Autodesk Inventor part; units mm, degrees
ref_plane "YZ Plane" through (0, 0, 0) normal (1, 0, 0) x (0, 1, 0)
ref_plane "XZ Plane" through (0, 0, 0) normal (0, 1, 0) x (-1, 0, 0)
ref_plane "XY Plane" through (0, 0, 0) normal (0, 0, 1) x (1, 0, 0)
sketch "Sketch1" plane through (0, 0, 0) normal (1, 0, 0) x (0, 1, 0)
  line L0 (0, 18.823) -> (0, -81.823)
  line L1 (-50.323, 0) -> (13.573, 0)
  line L2 (0, 0) -> (0, -63)
  line L3 (0, -63) -> (-28, -63)
  line L4 (-28, -63) -> (-28, -24.33)
  line L5 (-28, -24.33) -> (-36.75, -24.33)
  line L6 (-36.75, -24.33) -> (-36.75, 0)
  line L7 (-36.75, 0) -> (0, 0)
  circle A0 centre (-16, -42.5) radius 1.575 construction
  line L8 (-35.988, -0.762) -> (-35.988, -23.568)
  line L9 (-35.988, -23.568) -> (-27.238, -23.568)
  line L10 (-27.238, -23.568) -> (-27.238, -62.238)
  line L11 (-27.238, -62.238) -> (-0.762, -62.238)
  line L12 (-0.762, -62.238) -> (-0.762, -0.762)
  line L13 (-0.762, -0.762) -> (-35.988, -0.762)
  line L14 (-41.195, 4.445) -> (-41.195, -28.775)
  line L15 (-41.195, -28.775) -> (-32.445, -28.775)
  line L16 (-32.445, -28.775) -> (-32.445, -67.445)
  line L17 (-32.445, -67.445) -> (4.445, -67.445)
  line L18 (4.445, -67.445) -> (4.445, 4.445)
  line L19 (4.445, 4.445) -> (-41.195, 4.445)
  line L20 (1.905, 1.905) -> (-29.905, 1.905) construction
  line L21 (-29.905, 1.905) -> (-29.905, -64.905) construction
  line L22 (-29.905, -64.905) -> (1.905, -64.905) construction
  line L23 (1.905, -64.905) -> (1.905, 1.905) construction
  dimension "d0" = 63
  dimension "d1" = 28
  dimension "d2" = 36.75
  dimension "d3" = 24.33
  dimension "d4" = 42.5
  dimension "d5" = 16
  dimension "d6" = 3.15
  dimension "d16" = 0.762
  dimension "d17" = 4.445
  dimension "d18" = 2.54
  dimension "d19" = 2.54
  dimension "d20" = 2.54
  dimension "d21" = 2.54
  dimension "d29" = 66.81
  dimension "d30" = 31.81
extrude "Extrusion1" add sketch "Sketch1" against normal blind 4.4958
hole "Hole1" at (0, -16, -42.5) direction (-1, 0, 0) diameter 3.15 end through all
hole "Hole2" at (0, 1.905, 1.905) at (0, -29.905, -64.905) direction (-1, 0, 0) diameter 2.6 end through all
equation "\"d20\" = d18"
equation "\"d21\" = d18"
properties part number "J010359" material "ACRYLIC, BLACK"
Check sheet for the modelled part. Datum: model origin and axes. Units: mm. A direction names the side the tool comes from. Round coordinates to 2 decimals unless told otherwise and drop trailing zeros. Order: outer loops, then holes, each group sorted by start corner. A loop starts at its lowest first (then second) coordinate and runs counter-clockwise, first axis right, second up. Notation, with made-up numbers: M 34.25,45.25 L 70.25,45.25 A27 ccw 70.25,78.25 Z; hole C -16,70 d5. An arc over 180 degrees is marked long. Answer in a Markdown table with one row per item.
(1) Section check C-C on x = -0.95. Record the boundary of the cut face in (y, z) (3 decimals).
Findings:
| item | result |
|---|---|
| outline | M -41.195,-28.775 L -32.445,-28.775 L -32.445,-67.445 L 4.445,-67.445 L 4.445,4.445 L -41.195,4.445 Z; hole M -35.988,-23.568 L -27.238,-23.568 L -27.238,-62.238 L -0.762,-62.238 L -0.762,-0.762 L -35.988,-0.762 Z; hole C -29.905,-64.905 d2.6; hole C 1.905,1.905 d2.6 |
(2) Material ranges on line 1 along Z through (x, y) = (-1.45, -17) (3 decimals); line 2 along Y through (x, z) = (-2.5, -9) (3 decimals); line 3 along Y through (x, z) = (-2.2, -29) (3 decimals), recorded low to high. Write a range as from..to.
Findings:
| item | result |
|---|---|
| line 1 | z = -67.445..-62.238, -0.762..4.445 |
| line 2 | y = -41.195..-35.988, -0.762..4.445 |
| line 3 | y = -32.445..-27.238, -0.762..4.445 |
(3) Set-up check for faces 1 (the flat face through (-2, -32.445, -48)), 2 (the flat face through (-2, -35.988, -12)), 3 (the flat face through (-2, -14, -67.445)): record each of +Z, -Z, +X, -X, +Y, -Y from which the full face is reachable in a straight line by a thin tool's end or side.
Findings:
| item | result |
|---|---|
| face 1 | -Z, +X, -X, -Y |
| face 2 | +X, -X |
| face 3 | -Z, +X, -X, +Y, -Y |
(4) Gauge pin test, flat end, axial feed: pin 1 (2 mm diameter, centred on x = -3, y = -38, fed in from -Z) (3 decimals). Record the tip position at first contact, or that the pin passes through.
Findings:
| item | result |
|---|---|
| pin 1 | stops at z = -28.775 |
(5) Section check A-A on z = -47. Record the boundary of the cut face in (x, y) (3 decimals), plus the area to 3 significant figures.
Findings:
| item | result |
|---|---|
| outline | M -4.496,-32.445 L 0,-32.445 L 0,-27.238 L -4.496,-27.238 Z; M -4.496,-0.762 L 0,-0.762 L 0,4.445 L -4.496,4.445 Z |
| area | 46.8 mm^2 |
(6) Draft check along Z on faces 4 (the flat face through (-2, -18, 4.445)), 5 (the flat face through (-2, -18, -0.762)), 6 (the flat face through (-2, -37, -28.775)). Enter one of: +Z half, -Z half, draft (parallel to the pull), parting line (faces both ways), or undercut.
Findings:
| item | result |
|---|---|
| face 4 | +Z half |
| face 5 | undercut |
| face 6 | -Z half |
(7) Section check B-B on y = -14. Record the boundary of the cut face in (x, z) (3 decimals), plus the area to 3 significant figures.
Findings:
| item | result |
|---|---|
| outline | M -4.496,-67.445 L 0,-67.445 L 0,-62.238 L -4.496,-62.238 Z; M -4.496,-0.762 L 0,-0.762 L 0,4.445 L -4.496,4.445 Z |
| area | 46.8 mm^2 |
